from build123d import *

# Parameters (mm, degrees)
F0_R     = 12
F0_R_2   = 9
F1_DEPTH = 30
F0_R_3   = 6.5
F2_DEPTH = 25
F0_R_4   = 2.9
F3_DEPTH = 17
F0_R_5   = 2.1
F4_DEPTH = 8
F5_R     = 1


with BuildPart() as f1:
    # F0 (on Top) → F1 (new body)
    with BuildSketch(Plane.XY):
        Circle(F0_R)
        Circle(F0_R_2, mode=Mode.SUBTRACT)
    extrude(amount=F1_DEPTH)

    # F0 (on Top) → F2 (join)
    with BuildSketch(Plane.XY):
        Circle(F0_R_2)
        Circle(F0_R_3, mode=Mode.SUBTRACT)
    extrude(amount=F2_DEPTH)

    # F0 (on Top) → F3 (join)
    with BuildSketch(Plane.XY):
        Circle(F0_R_3)
        Circle(F0_R_4, mode=Mode.SUBTRACT)
    extrude(amount=F3_DEPTH)

    # F0 (on Top) → F4 (join)
    with BuildSketch(Plane.XY):
        Circle(F0_R_4)
        Circle(F0_R_5, mode=Mode.SUBTRACT)
    extrude(amount=F4_DEPTH)

    # F5
    f5_edges = [f1.edges().sort_by_distance(p)[0] for p in [
        (-12, 0, 0),
    ]]
    fillet(f5_edges, radius=F5_R)


solid = f1.part
Build history of the part. All positions in model axes, mm. A direction names the side the tool comes from. Give positions to 0.01 mm unless a question says otherwise; leave off trailing zeros. Write each loop counter-clockwise with the first axis right and the second up, starting at its lowest first coordinate (ties: lowest second). Pieces come first, ordered by that corner, then holes. Notation, with made-up numbers: (4, 28.5) - (27, 28.5) arc R24 cw to (27, 49.5) - close; hole circle Ø2 at (80.5, 53). An arc over 180 degrees is marked (long way). Use one line per item in the form item = value. Start each with the question number.
1. Two-plate mould, pull along X, no slides. Class faces 1 (the face through (-5.158, -3.955, 20.944)), 2 (the face through (-0.2, -2.3, 0)), 3 (the face through (-11.99, 0.53, 15.3)): released by +X, released by -X, zero draft, split by the parting line, or undercut.
2. 3-axis set-ups, long thin cutter, end or side, ignore diameter. For faces 4 (the face through (-1.172, 8.923, 27.465)), 5 (the face through (2.003, 0.631, 3.944)): which of +Z, -Z, +X, -X, +Y, -Y reach the whole face in a straight line?
3. Probe line 1 (Y direction, x = 0, z = 20); line 2 (Y direction, x = 0, z = 15.25); line 3 (X direction, y = -3.25, z = 22). List the from-to ranges inside material, lowest first. Write a range as [from, to].
4. Drop flat-ended pins along their axis: pin 1 Ø5.5 at (x, y) = (4, -2.5) entering from +Z; pin 2 Ø4 at (x, z) = (-6, 9.5) entering from -Y; pin 3 Ø3 at (y, z) = (-7, 17) entering from +X; pin 4 Ø4 at (x, y) = (0, 0) entering from -Z. Give the stop position or say it passes through.
5. Band-saw the part on A-A on y = 0. Write the cut outline in (x, z), plus the area to 3 significant figures.
6. Band-saw the part on C-C on z = 4.25. Write the cut outline in (x, y), plus the area to 3 significant figures.
Conclusion:
q1.face_1 = undercut
q1.face_2 = zero draft
q1.face_3 = split by the parting line
q2.face_4 = +Z
q2.face_5 = +Z, -Z
q3.line_1 = [-12, -6.5], [6.5, 12]
q3.line_2 = [-12, -2.9], [2.9, 12]
q3.line_3 = [-11.55, -5.63], [5.63, 11.55]
q4.pin_1 = 25
q4.pin_2 = -11.31
q4.pin_3 = 10.67
q4.pin_4 = through
q5.outline = (-12, 1) arc R1 ccw to (-11, 0) - (-2.1, 0) - (-2.1, 8) - (-2.9, 8) - (-2.9, 17) - (-6.5, 17) - (-6.5, 25) - (-9, 25) - (-9, 30) - (-12, 30) - close; (2.1, 0) - (11, 0) arc R1 ccw to (12, 1) - (12, 30) - (9, 30) - (9, 25) - (6.5, 25) - (6.5, 17) - (2.9, 17) - (2.9, 8) - (2.1, 8) - close
q5.area = 440 mm²
q6.outline = circle Ø24 at (0, 0); hole circle Ø4.2 at (0, 0)
q6.area = 439 mm²
